```python
from build123d import *

# Parameters (mm, degrees)
SKETCH3_W           = 6
SKETCH3_H           = 5
BOSS_EXTRUDE6_DEPTH = 6
CUT_EXTRUDE4_DEPTH  = 6
CUT_EXTRUDE5_DEPTH  = 3


with BuildPart() as part:
    # Sketch3 → Boss-Extrude6 (new body)
    with BuildSketch(Plane.XY):
        with Locations((3, 2.5)):
            Rectangle(SKETCH3_W, SKETCH3_H)
    extrude(amount=BOSS_EXTRUDE6_DEPTH)

    # Sketch7 → Cut-Extrude4 (cut)
    with BuildSketch(Plane.ZY):
        Polygon((0, 5), (6, 4), (6, 5), align=None)
    extrude(amount=-CUT_EXTRUDE4_DEPTH, mode=Mode.SUBTRACT)

    # Sketch8 → Cut-Extrude5 (cut)
    with BuildSketch(Plane.ZY):
        Polygon((0, 5), (6, 4), (6, 3), (0, 1), align=None)
    extrude(amount=-CUT_EXTRUDE5_DEPTH, mode=Mode.SUBTRACT)


solid = part.part
```
Geometry check sheet. Reference: the model listing, model coordinates, mm. A direction names the side the tool comes from. Round coordinates to 2 decimals unless told otherwise and drop trailing zeros. Loops run counter-clockwise (first coordinate to the right, second up) from the corner with the lowest first, then second, coordinate; pieces in that order, holes last. Notation, with made-up numbers: (46.25, 56) - (84.25, 56) arc R27 cw to (84.25, 82) - close; hole circle Ø10 at (19.25, 31). An arc over 180 degrees is marked (long way). Write item = value, one per line. Start each with the question number.
1. Set-up check for faces 1 (the face through (0, 1, 4)), 2 (the face through (3, 3, 2)): record each of +Z, -Z, +X, -X, +Y, -Y from which the full face is reachable in a straight line by a thin tool's end or side.
2. Section check B-B on y = 1.25. Enter the section's corners in (x, z), then the cut area to 4 significant figures.
3. Section check C-C on x = 0.4. Enter the section's corners in (y, z).
4. Depth check by flat-ended pin: pin 1 (1 mm diameter, centred on y = 3, z = 1, fed in from -X). Enter the tip coordinate at first touch or a pass-through.
5. Section check D-D on x = 4.6. Enter the section's corners in (y, z).
6. Thickness scan on line 1 (X direction, y = 3.7, z = 2.25); line 2 (Y direction, x = 5.85, z = 1); line 3 (Y direction, x = 5.5, z = 3.75) (3 decimals). Record the ranges inside material, lowest first.
7. Section check A-A on z = 4.5. Enter the section's corners in (x, y), then the cut area to 4 significant figures.
Working result:
q1.face_1 = +Z, -Z, -X, +Y, -Y
q1.face_2 = -Z, -X, +Y
q2.outline = (0, 0.75) - (3, 0.75) - (3, 0) - (6, 0) - (6, 6) - (0, 6) - close
q2.area = 33.75 mm^2
q3.outline = (0, 0) - (1, 0) - (3, 6) - (0, 6) - close
q4.pin_1 = 3
q5.outline = (0, 0) - (5, 0) - (4, 6) - (0, 6) - close
q6.line_1 = 3 to 6
q6.line_2 = 0 to 4.83
q6.line_3 = 0 to 4.375
q7.outline = (0, 0) - (6, 0) - (6, 4.25) - (3, 4.25) - (3, 2.5) - (0, 2.5) - close
q7.area = 20.25 mm^2
